```python
from build123d import *

# Parameters (mm, degrees)
ESTRUSIONE_ESTRUSIONE1_DEPTH = 10
SCHIZZO2_W                   = 100
SCHIZZO2_H                   = 35
ESTRUSIONE_ESTRUSIONE2_DEPTH = 1
SCHIZZO3_R                   = 4.5
SCHIZZO4_R                   = 3


with BuildPart() as part:
    # Schizzo1 → Estrusione-Estrusione1 (new body)
    with BuildSketch(Plane.XY):
        Polygon((-60, 60), (-60, 0), (0, 0), (0, -10), (60, -10), (60, 0.1203125), (60, 60), align=None)
    extrude(amount=ESTRUSIONE_ESTRUSIONE1_DEPTH)

    # Schizzo2 → Estrusione-Estrusione2 (add)
    with BuildSketch(Plane.XY.offset(10)):
        with Locations((0, 30)):
            Rectangle(SCHIZZO2_W, SCHIZZO2_H)
    extrude(amount=ESTRUSIONE_ESTRUSIONE2_DEPTH)

    # Schizzo3 → Loft1 section 0
    with BuildSketch(Plane.XY.offset(10)):
        with Locations((35, 0)):
            Circle(SCHIZZO3_R)
    # Schizzo4 → Loft1 section 1
    with BuildSketch(Plane.XY.offset(20)):
        with Locations((35, 0)):
            Circle(SCHIZZO4_R)
    loft()


solid = part.part
```
Model file for the job. Use its own axes, mm. A direction names the side the tool comes from. Give positions to 0.01 mm unless a question says otherwise; leave off trailing zeros. Write each loop counter-clockwise with the first axis right and the second up, starting at its lowest first coordinate (ties: lowest second). Pieces come first, ordered by that corner, then holes. Notation, with made-up numbers: (36.25, -27.5) - (74.25, -27.5) arc R17 cw to (74.25, -0.5) - close; hole circle Ø7 at (26.5, -21.5). An arc over 180 degrees is marked (long way). One line per question, with ' | ' between items. Start each with the question number.
(1) Wall check: line 1 along Z through (x, y) = (4, -7); line 2 along Z through (x, y) = (18, 22); line 3 along Y through (x, z) = (-16.5, 10.75). Give the ranges that are in metal, low to high. Write a range as from..to.
(2) Slice it at B-B on y = 35. Write the cut outline in (x, z), plus the area to 3 significant figures.
(3) Pin check, flat tips, straight feed: P1, Ø17.5, axis at x = 21.5, y = 33.5, coming from the +Z side; P2, Ø10, axis at x = -33, z = 8.5, coming from the -Y side; P3, Ø3, axis at y = 0.5, z = 12, coming from the +X side; P4, Ø10, axis at y = 44.5, z = 16.5, coming from the +X side. Stop position of each tip, or through.
(4) Slice it at D-D on x = 35. Write the cut outline in (y, z), plus the area to 3 significant figures.
(5) Slice it at A-A on x = 3.5. Write the cut outline in (y, z).
(6) Slice it at C-C on z = 5.25. Write the cut outline in (x, y).
(7) 3-axis set-ups, long thin cutter, end or side, ignore diameter. For faces 1 (the face through (0, -5, 5)), 2 (the face through (30, -10, 5)), 3 (the face through (-1, 10, 10)): which of +Z, -Z, +X, -X, +Y, -Y reach the whole face in a straight line?
Results below:
1) line 1: 0..10 | line 2: 0..11 | line 3: 12.5..47.5
2) outline: (-60, 0) - (60, 0) - (60, 10) - (50, 10) - (50, 11) - (-50, 11) - (-50, 10) - (-60, 10) - close | area: 1,300 mm^2
3) P1: z = 11 | P2: y = 0 | P3: x = 39.42 | P4: through
4) outline: (-10, 0) - (60, 0) - (60, 10) - (47.5, 10) - (47.5, 11) - (12.5, 11) - (12.5, 10) - (4.5, 10) - (3, 20) - (-3, 20) - (-4.5, 10) - (-10, 10) - close | area: 810 mm^2
5) outline: (-10, 0) - (60, 0) - (60, 10) - (47.5, 10) - (47.5, 11) - (12.5, 11) - (12.5, 10) - (-10, 10) - close
6) outline: (-60, 0) - (0, 0) - (0, -10) - (60, -10) - (60, 60) - (-60, 60) - close
7) face 1: +Z, -Z, -X, -Y | face 2: +Z, -Z, +X, -X, -Y | face 3: +Z
